Can you work these out from the model? Positions are in its coordinate system, mm. A direction names the side the tool comes from. Round coordinates to 2 decimals unless told otherwise and drop trailing zeros. Order: outer loops, then holes, each group sorted by start corner. A loop starts at its lowest first (then second) coordinate and runs counter-clockwise, first axis right, second up.
from build123d import *

# Parameters (mm, degrees)
F0_W     = 11.1455010677
F0_H     = 11.1455010677
F1_DEPTH = 25


with BuildPart() as f1:
    # F0 (on Front) → F1 (new body)
    with BuildSketch(Plane.XZ):
        Polygon((3.4639391611, 41.4549691979), (22.3714864994, 41.4549691979), (22.3714864994, 52.6004702657), align=None)
        with Locations((27.9442370333, 47.0277197318)):
            Rectangle(F0_W, F0_H)
        Polygon((33.5169875672, 23.542555845), (33.5169875672, 41.4549691979), (22.3714864994, 41.4549691979), align=None)
        Polygon((33.5169875672, 52.6004702657), (33.5169875672, 41.4549691979), (52.4245357128, 52.6004702657), align=None)
        Polygon((22.3714864994, 52.6004702657), (33.5169875672, 52.6004702657), (22.3714864994, 70.1275136257), align=None)
    extrude(amount=F1_DEPTH)


solid = f1.part
(1) Please list where these lines run through material, in increasing order: probe 1 along X at (y, z) = (-13, 60); probe 2 along X at (y, z) = (-14, 53); probe 3 along Z at (x, y) = (44, -3).
(2) I want a section at C-C, the plane x = 20.5. List the corners of the cut face in (y, z) for me.
(3) I want a section at A-A, the plane y = -15.5. List the corners of the cut face in (x, z) for me.
(4) I want a section at B-B, the plane z = 59. List the corners of the cut face in (x, y) for me, plus the area to 3 significant figures.
(5) I'm going to push flat-ended pins straight in: pin 1 Ø4 at (y, z) = (-10.5, 29) entering from +X; pin 2 Ø4 at (y, z) = (-7.5, 58.5) entering from +X; pin 3 Ø5.5 at (y, z) = (-13, 64.5) entering from -X. Where does each tip first touch, or does it pass through?
(6) On a 3-axis mill with a long thin cutter (end or side, diameter ignored), from which of +Z, -Z, +X, -X, +Y, -Y can I reach the whole of each face in a straight line? I mean faces 1 (the face through (43, -12, 52.6)), 2 (the face through (13, -12, 41.455)), 3 (the face through (33.517, -12, 32)), 4 (the face through (22.371, -12, 61)). Say none if no direction works.
Ans:
1. probe 1: x = 22.37 to 28.81
1. probe 2: x = 22.37 to 33.26
1. probe 3: z = 47.63 to 52.6
2. outline: (-25, 41.45) - (0, 41.45) - (0, 51.5) - (-25, 51.5) - close
3. outline: (3.46, 41.45) - (22.37, 41.45) - (33.52, 23.54) - (33.52, 41.45) - (52.42, 52.6) - (33.52, 52.6) - (22.37, 70.13) - (22.37, 52.6) - close
4. outline: (22.37, -25) - (29.45, -25) - (29.45, 0) - (22.37, 0) - close
4. area: 177 mm2
5. pin 1: stops at x = 33.52
5. pin 2: stops at x = 31.04
5. pin 3: stops at x = 22.37
6. face 1: +Z, +X, +Y, -Y
6. face 2: -Z, -X, +Y, -Y
6. face 3: -Z, +X, +Y, -Y
6. face 4: +Z, -X, +Y, -Y
